Geometry check sheet. Reference: the model listing, model coordinates, mm. A direction names the side the tool comes from. Give positions to 0.01 mm unless a question says otherwise; leave off trailing zeros. Loops run counter-clockwise (first coordinate to the right, second up) from the corner with the lowest first, then second, coordinate; pieces in that order, holes last. Notation, with made-up numbers: (-27.75, 81.5) - (-11.75, 81.5) arc R19 cw to (-11.75, 108.5) - close; hole circle Ø8 at (22, -5.75). An arc over 180 degrees is marked (long way). Use a Markdown table: item, result. Add a question column.
1. Set-up check for faces 4 (the flat face through (5, -5, 1)), 5 (the flat face through (-6, -5, 1)): record each of +Z, -Z, +X, -X, +Y, -Y from which the full face is reachable in a straight line by a thin tool's end or side.
2. Cross-section at C-C on x = 1. Enter the section's corners in (y, z), and give its area (4 significant figures).
3. Material ranges on L1, parallel to X at y = -5.25, z = 1.2; L2, parallel to Z at x = -3.5, y = -5.75; L3, parallel to X at y = -8.25, z = 1.9, recorded low to high.
4. Cross-section at B-B on y = -4. Enter the section's corners in (x, z), and give its area (3 significant figures).
5. Cross-section at A-A on z = 1.4. Enter the section's corners in (x, y), and give its area (3 significant figures).
6. Cross-section at D-D on z = 0.15. Enter the section's corners in (x, y).
7. Draft check along X on faces 1 (the flat face through (6, -5, 1)), 2 (the flat face through (-1.3, 0, 0.5)), 3 (the flat face through (-5, -5, 1)). Enter one of: pulls with the +X half, pulls with the -X half, needs draft (parallel to the pull), parting line crosses it, or undercut.
from build123d import *

# Parameters (mm, degrees)
F0_W     = 12
F0_H     = 9
F1_DEPTH = 2
F2_W     = 10
F2_H     = 9
F3_DEPTH = 1.2
F4_SIZE  = 0.3


with BuildPart() as f1:
    # F0 (on Top) → F1 (new body)
    with BuildSketch(Plane.XY):
        with Locations((0, -4.5)):
            Rectangle(F0_W, F0_H)
    extrude(amount=F1_DEPTH)

    # F2 (on face) → F3 (cut)
    with BuildSketch(Plane.XY.offset(2)):
        with Locations((0, -4.5)):
            Rectangle(F2_W, F2_H)
    extrude(amount=-F3_DEPTH, mode=Mode.SUBTRACT)

    # F4
    f4_edges = [f1.edges().sort_by_distance(p)[0] for p in [
        (-6, -4.5, 2),
        (6, -4.5, 2),
        (6, -4.5, 0),
        (-6, -4.5, 0),
        (0, 0, 0),
        (-6, 0, 1),
        (-5.5, 0, 2),
        (5.5, 0, 2),
        (6, 0, 1),
    ]]
    chamfer(f4_edges, length=F4_SIZE)


solid = f1.part
Values found:
| question | item | result |
|---|---|---|
| 1 | face 4 | +Z, +Y, -Y |
| 1 | face 5 | +Z, -Z, -X, +Y, -Y |
| 2 | outline | (-9, 0) - (-0.3, 0) - (0, 0.3) - (0, 0.8) - (-9, 0.8) - close |
| 2 | area | 7.155 mm2 |
| 3 | L1 | x = -6 to -5, 5 to 6 |
| 3 | L2 | z = 0 to 0.8 |
| 3 | L3 | x = -5.8 to -5, 5 to 5.8 |
| 4 | outline | (-6, 0.3) - (-5.7, 0) - (5.7, 0) - (6, 0.3) - (6, 1.7) - (5.7, 2) - (5, 2) - (5, 0.8) - (-5, 0.8) - (-5, 2) - (-5.7, 2) - (-6, 1.7) - close |
| 4 | area | 11.8 mm2 |
| 5 | outline | (-6, -9) - (-5, -9) - (-5, 0) - (-5.7, 0) - (-6, -0.3) - close; (5, -9) - (6, -9) - (6, -0.3) - (5.7, 0) - (5, 0) - close |
| 5 | area | 17.9 mm2 |
| 6 | outline | (-5.85, -9) - (5.85, -9) - (5.85, -0.3) - (5.7, -0.15) - (-5.7, -0.15) - (-5.85, -0.3) - close |
| 7 | face 1 | pulls with the +X half |
| 7 | face 2 | needs draft |
| 7 | face 3 | undercut |
